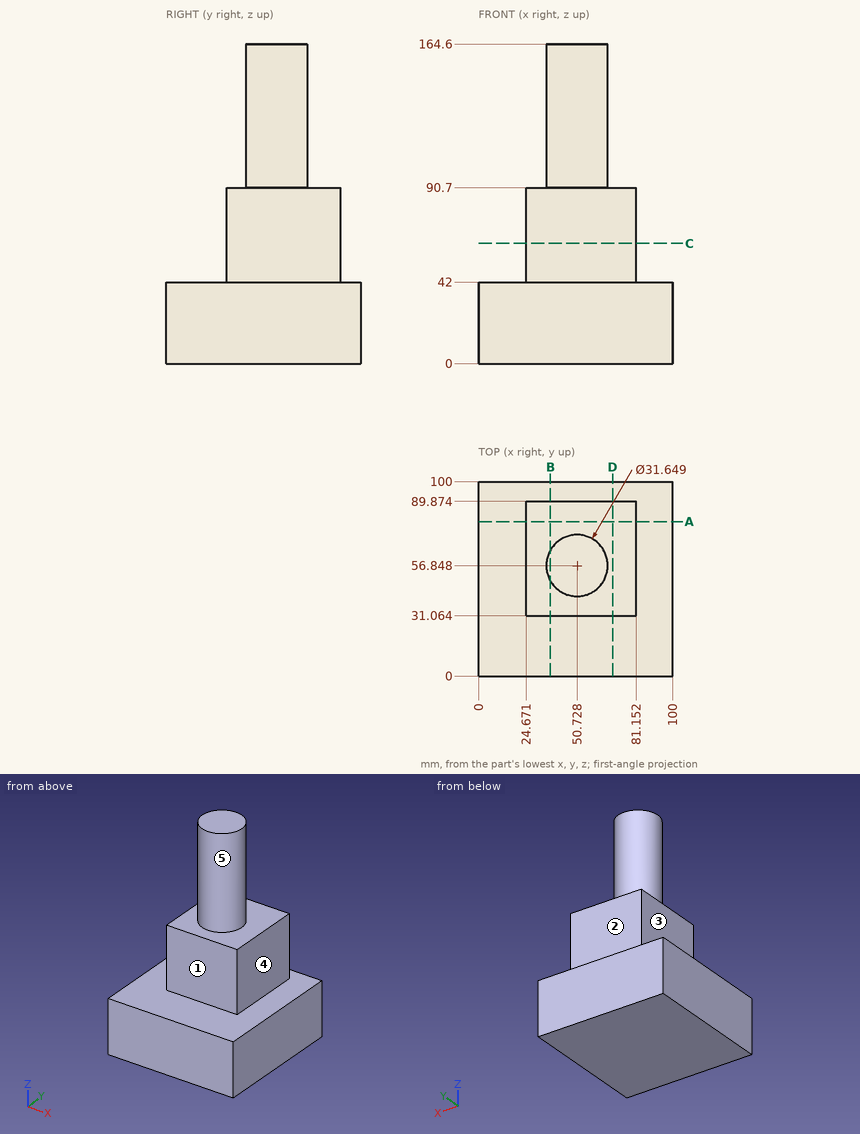
The figure shows three views and two pictorial views of one solid part (mm, origin at its lowest corner). Answer the questions. A direction names the side the tool comes from. Coordinates: 2 decimals unless noted, no trailing zeros. Loops run counter-clockwise (first coordinate to the right, second up) from the corner with the lowest first, then second, coordinate; pieces in that order, holes last.
1) Find the intervals of material crossed by L1, parallel to Z at x = 61, y = 84.5; L2, parallel to Z at x = 16, y = 46.5; L3, parallel to Y at x = 61.5, z = 71 (1 decimal), in increasing order.
2) Find section B-B on x = 37. Write down the section's boundary in (y, z) (1 decimal), then the cut area to 3 significant figures.
3) Flat-ended cylindrical pins translate along their axes: pin 1 Ø24.5 at (y, z) = (60, 66.5) entering from +X; pin 2 Ø10 at (x, y) = (41.5, 82.5) entering from -Z; pin 3 Ø6 at (y, z) = (46, 135) entering from -X; pin 4 Ø1.5 at (x, y) = (22.5, 47.5) entering from +Z. Find the tip coordinate at first contact, or state that the pin passes through.
4) A tool of negligible diameter and unlimited length cuts with its end or side. For the marked faces 1, 2, 3, 4 and 5, from which of +Z, -Z, +X, -X, +Y, -Y can it reach the whole face along a straight path? Write none if from no direction.
5) Find section C-C on z = 62. Write down the section's boundary in (x, y) (1 decimal).
6) Find section D-D on x = 69. Write down the section's boundary in (y, z) (1 decimal).
7) Find section A-A on y = 79.5. Write down the section's boundary in (x, z), then the cut area to 3 significant figures.
Values:
1. L1: z = 0 to 90.7
1. L2: z = 0 to 42
1. L3: y = 31.1 to 89.9
2. outline: (0, 0) - (100, 0) - (100, 42) - (89.9, 42) - (89.9, 90.7) - (64.7, 90.7) - (64.7, 164.6) - (49, 164.6) - (49, 90.7) - (31.1, 90.7) - (31.1, 42) - (0, 42) - close
2. area: 8,230 mm2
3. pin 1: stops at x = 81.15
3. pin 2: stops at z = 0
3. pin 3: stops at x = 36.99
3. pin 4: stops at z = 42
4. face 1: +Z, +X, -X, -Y
4. face 2: +Z, +X, -X, +Y
4. face 3: +Z, -X, +Y, -Y
4. face 4: +Z, +X, +Y, -Y
4. face 5: +Z
5. outline: (24.7, 31.1) - (81.2, 31.1) - (81.2, 89.9) - (24.7, 89.9) - close
6. outline: (0, 0) - (100, 0) - (100, 42) - (89.9, 42) - (89.9, 90.7) - (31.1, 90.7) - (31.1, 42) - (0, 42) - close
7. outline: (0, 0) - (100, 0) - (100, 42) - (81.15, 42) - (81.15, 90.7) - (24.67, 90.7) - (24.67, 42) - (0, 42) - close
7. area: 6,950 mm2
